Part model, mm, in its own coordinate system. Coordinates: 2 decimals unless noted, no trailing zeros.
```python
from build123d import *

# Parameters (mm, degrees)
CROQUIS1_W                                           = 410
CROQUIS1_H                                           = 90
SALIENTE_EXTRUIR1_DEPTH                              = 10
CHAFL_N1_SIZE                                        = 5
AVELLANADO_PARA_TORNILLO_CON_CABEZA_AVEL_D           = 4.5
AVELLANADO_PARA_TORNILLO_CON_CABEZA_AVEL_CSINK_D     = 9.18
AVELLANADO_PARA_TORNILLO_CON_CABEZA_AVEL_CSINK_ANGLE = 90
AVELLANADO_PARA_TORNILLO_CON_CABEZA_2_D              = 4.5
AVELLANADO_PARA_TORNILLO_CON_CABEZA_2_CSINK_D        = 9.18
AVELLANADO_PARA_TORNILLO_CON_CABEZA_2_CSINK_ANGLE    = 90
AVELLANADO_PARA_TORNILLO_CON_CABEZA_3_D              = 4.5
AVELLANADO_PARA_TORNILLO_CON_CABEZA_3_CSINK_D        = 9.18
AVELLANADO_PARA_TORNILLO_CON_CABEZA_3_CSINK_ANGLE    = 90
AVELLANADO_PARA_TORNILLO_CON_CABEZA_4_D              = 4.5
AVELLANADO_PARA_TORNILLO_CON_CABEZA_4_CSINK_D        = 9.18
AVELLANADO_PARA_TORNILLO_CON_CABEZA_4_CSINK_ANGLE    = 90


with BuildPart() as part:
    # Croquis1 → Saliente-Extruir1 (new body)
    with BuildSketch(Plane(origin=(0, 0, 0), x_dir=(1, 0, 0), z_dir=(0, 1, 0))):
        with Locations((205, 0)):
            Rectangle(CROQUIS1_W, CROQUIS1_H)
    extrude(amount=SALIENTE_EXTRUIR1_DEPTH)

    # Chaflán1
    chafl_n1_edges = [part.edges().sort_by_distance(p)[0] for p in [
        (410, 5, 45),
        (0, 5, 45),
        (0, 5, -45),
        (410, 5, -45),
    ]]
    chamfer(chafl_n1_edges, length=CHAFL_N1_SIZE)

    # Avellanado para tornillo con cabeza avel (through all)
    with Locations(Plane(origin=(0, 0, 0), x_dir=(-1, 0, 0), z_dir=(0, -1, 0))):
        with Locations((-15, -25), (-45, 25), (-45, -25), (-15, 25)):
            CounterSinkHole(AVELLANADO_PARA_TORNILLO_CON_CABEZA_AVEL_D / 2, AVELLANADO_PARA_TORNILLO_CON_CABEZA_AVEL_CSINK_D / 2, counter_sink_angle=AVELLANADO_PARA_TORNILLO_CON_CABEZA_AVEL_CSINK_ANGLE)

    # Avellanado para tornillo con cabeza  2 (through all)
    with Locations(Plane(origin=(0, 0, 0), x_dir=(-1, 0, 0), z_dir=(0, -1, 0))):
        with Locations((-235, 38), (-235, 6), (-235, -6), (-235, -38)):
            CounterSinkHole(AVELLANADO_PARA_TORNILLO_CON_CABEZA_2_D / 2, AVELLANADO_PARA_TORNILLO_CON_CABEZA_2_CSINK_D / 2, counter_sink_angle=AVELLANADO_PARA_TORNILLO_CON_CABEZA_2_CSINK_ANGLE)

    # Avellanado para tornillo con cabeza  3 (through all)
    with Locations(Plane(origin=(0, 0, 0), x_dir=(-1, 0, 0), z_dir=(0, -1, 0))):
        with Locations((-290, 15), (-310, -15), (-310, 15), (-290, -15)):
            CounterSinkHole(AVELLANADO_PARA_TORNILLO_CON_CABEZA_3_D / 2, AVELLANADO_PARA_TORNILLO_CON_CABEZA_3_CSINK_D / 2, counter_sink_angle=AVELLANADO_PARA_TORNILLO_CON_CABEZA_3_CSINK_ANGLE)

    # Avellanado para tornillo con cabeza  4 (through all)
    with Locations(Plane(origin=(0, 0, 0), x_dir=(-1, 0, 0), z_dir=(0, -1, 0))):
        with Locations((-270, 32.5), (-350, -32.5), (-350, 32.5), (-270, -32.5)):
            CounterSinkHole(AVELLANADO_PARA_TORNILLO_CON_CABEZA_4_D / 2, AVELLANADO_PARA_TORNILLO_CON_CABEZA_4_CSINK_D / 2, counter_sink_angle=AVELLANADO_PARA_TORNILLO_CON_CABEZA_4_CSINK_ANGLE)


solid = part.part
```
Q1. Probe line 1 (X direction, y = 7, z = 25); line 2 (Z direction, x = 350, y = 5.5); line 3 (Z direction, x = 15, y = 4.75). List the from-to ranges inside material, lowest first.
Q2. Drop flat-ended pins along their axis: P1, Ø2.5, axis at x = 45, z = 25, coming from the +Y side; P2, Ø7, axis at x = 235, z = 38, coming from the -Y side. Give the stop position or say it passes through.
Q3. Mould opens along X. For faces 1 (the conical face through (237.25, 2.23, 37.29)), 2 (the flat face through (0, 5, 1)), 3 (the flat face through (202, 5, -45)), 4 (the flat face through (410, 5, 1)) say: released by +X, released by -X, zero draft, split by the parting line, or undercut.
Checked values:
1. line 1: x = 0 to 12.75, 17.25 to 42.75, 47.25 to 410
1. line 2: z = -45 to -34.75, -30.25 to 30.25, 34.75 to 45
1. line 3: z = -45 to -27.25, -22.75 to 22.75, 27.25 to 45
2. P1: passes through
2. P2: stops at y = 1.09
3. face 1: undercut
3. face 2: released by -X
3. face 3: zero draft
3. face 4: released by +X
